For this review, take the finished solid that the model builds, in its own axes (mm). Face numbers are marked on the shaded views. Give positions to 0.01 mm unless a question says otherwise; leave off trailing zeros. Loops run counter-clockwise (first coordinate to the right, second up) from the corner with the lowest first, then second, coordinate; pieces in that order, holes last. Notation, with made-up numbers: (17.5, -28) - (66.5, -28) arc R27 ccw to (66.5, 9) - close; hole circle Ø11 at (13, 50.25). An arc over 180 degrees is marked (long way). Answer in a Markdown table with one row per item.
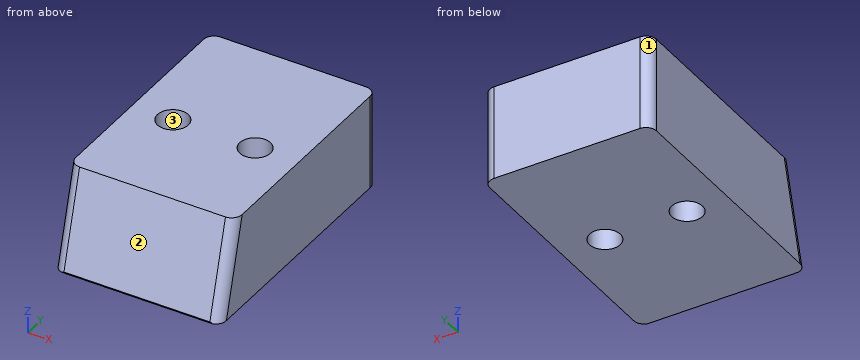
Autodesk Inventor part; units mm, degrees
ref_plane "YZ Plane" through (0, 0, 0) normal (1, 0, 0) x (0, 1, 0)
ref_plane "XZ Plane" through (0, 0, 0) normal (0, 1, 0) x (-1, 0, 0)
ref_plane "XY Plane" through (0, 0, 0) normal (0, 0, 1) x (1, 0, 0)
sketch "Szkic1" plane through (0, 0, 0) normal (0, 0, 1) x (1, 0, 0)
  line L0 (-10.8514, 21.0596) -> (5.3486, 21.0596)
  line L1 (5.3486, 21.0596) -> (5.3486, -3.9404)
  line L2 (5.3486, -3.9404) -> (-10.8514, -3.9404)
  line L3 (-10.8514, -3.9404) -> (-10.8514, 21.0596)
  point P0 (0, 0)
  dimension "d0" = 16.2
  dimension "d1" = 25
extrude "Wyciągnięcie proste1" add sketch "Szkic1" along normal blind 9.2
sketch "Szkic2" plane through (0, 0, 9.2) normal (0, 0, 1) x (1, 0, 0)
  line L0 (5.3486, 21.0596) -> (-10.8514, 21.0596)
  line L1 (-10.8514, 21.0596) -> (-10.8514, -3.9404)
  line L2 (-10.8514, -3.9404) -> (5.3486, -3.9404)
  line L3 (5.3486, -3.9404) -> (5.3486, 21.0596)
  point P0 (0, 0)
  point P1 (-6.8514, 8.5596)
  point P2 (1.1486, 8.5596)
  dimension "d4" = 12.5
  dimension "d5" = 12.5
  dimension "d6" = 4
  dimension "d7" = 4.2
hole "Otwór1" at (-6.8514, 8.5596, 9.2) at (1.1486, 8.5596, 9.2) direction (0, 0, -1) diameter 3 end through all
chamfer "Faza3" distance 2.5 distance2 9.1 1 edges at (-2.7514, -3.9404, 9.2) measured on face at (-1.6837, 17.3356, 9.2)
fillet "Zaokrąglenie1" radius 1 4 edges at (-10.8514, 21.0596, 4.6) (5.3486, -2.6904, 4.65) (-10.8514, -2.6904, 4.65) (5.3486, 21.0596, 4.6)
properties part number "3DP_ABS_X_Axis_IGUS_Cable_Chain_Mount"
1. We need section C-C, the plane z = 6.25. Count the separate pieces of the cut face and the enclosed holes in it, and give its area (3 significant figures).
Values:
| item | result |
|---|---|
| separate pieces | 1 |
| enclosed holes | 2 |
| area | 363 mm^2 |
2. Mouldability with a two-part tool opening along X and no side actions: class the marked faces 1, 2 and 3 as released by +X, released by -X, zero draft, split by the parting line, or undercut.
Values:
| item | result |
|---|---|
| face 1 | released by -X |
| face 2 | zero draft |
| face 3 | undercut |
3. We need section B-B, the plane x = -9.25. Give the boundary of the cut face in (y, z), and give its area (3 significant figures).
Values:
| item | result |
|---|---|
| outline | (-3.94, 0) - (21.06, 0) - (21.06, 9.2) - (-1.44, 9.2) - (-3.94, 0.1) - close |
| area | 219 mm^2 |
4. Wall thickness on line 1 (X direction, y = 7.5, z = 2.75); line 2 (Y direction, x = -7, z = 4.75); line 3 (Y direction, x = -7.5, z = 7.5): over which ranges is each line inside the solid? List them lowest first. Write a range as [from, to].
Values:
| item | result |
|---|---|
| line 1 | x = [-10.85, -7.91], [-5.79, 0.09], [2.21, 5.35] |
| line 2 | y = [-2.66, 7.07], [10.05, 21.06] |
| line 3 | y = [-1.91, 7.21], [9.91, 21.06] |
5. We need section A-A, the plane x = 0. Give the boundary of the cut face in (y, z).
Values:
| item | result |
|---|---|
| outline | (-3.94, 0) - (7.59, 0) - (7.59, 9.2) - (-1.44, 9.2) - (-3.94, 0.1) - close; (9.52, 0) - (21.06, 0) - (21.06, 9.2) - (9.52, 9.2) - close |
6. Clearance check with a flat-ended pin moving along its axis: pin 1 (5 mm diameter, centred on x = -7.5, z = 7.5, fed in from -Y). State where the tip first meets the part, or that it passes through.
Values:
| item | result |
|---|---|
| pin 1 | stops at y = -2.59 |
7. We need section D-D, the plane x = 2. Give the boundary of the cut face in (y, z).
Values:
| item | result |
|---|---|
| outline | (-3.94, 0) - (7.32, 0) - (7.32, 9.2) - (-1.44, 9.2) - (-3.94, 0.1) - close; (9.79, 0) - (21.06, 0) - (21.06, 9.2) - (9.79, 9.2) - close |
